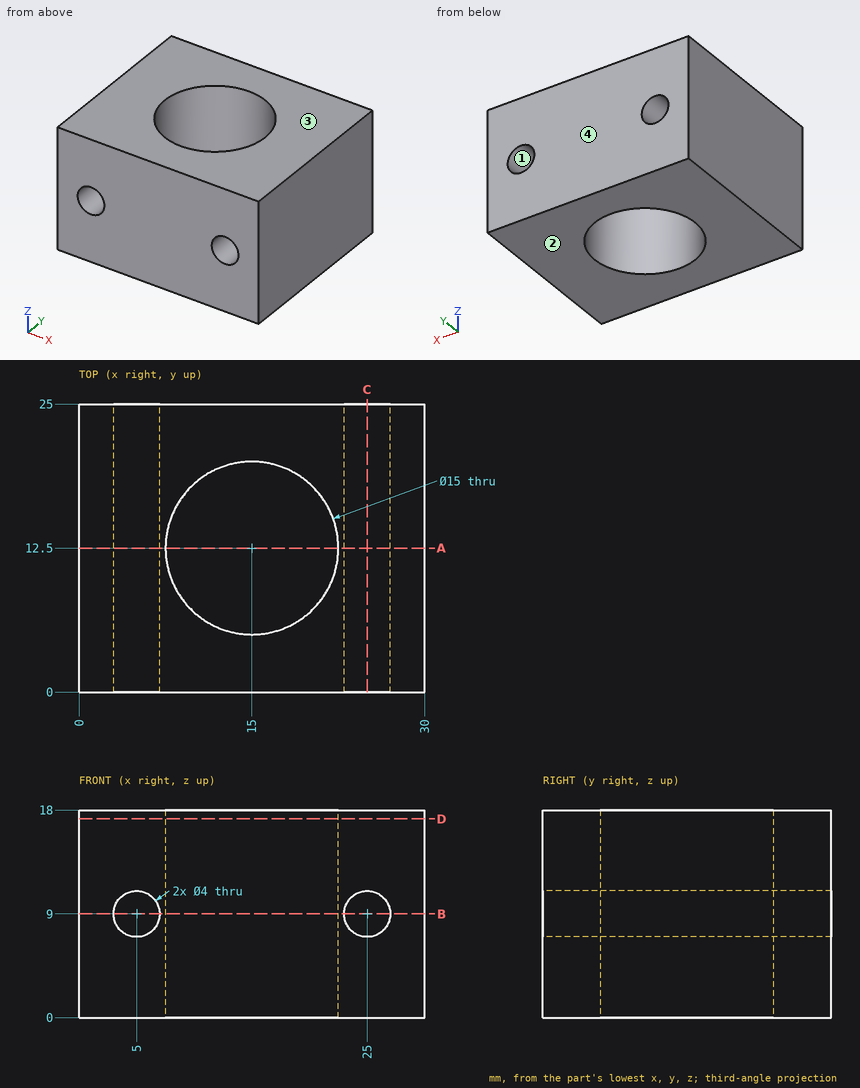
Design review of the part shown in the three views and the two pictorial views. Dimensions are in mm from the part's minimum x, y and z. Coordinates: 2 decimals unless noted, no trailing zeros. Loops run counter-clockwise (first coordinate to the right, second up) from the corner with the lowest first, then second, coordinate; pieces in that order, holes last. Notation, with made-up numbers: (42, 75) - (87, 75) arc R19 ccw to (87, 106) - close; hole circle Ø2 at (-39, 40.5). An arc over 180 degrees is marked (long way). Use a Markdown table: item, result. Add a question column.
Item 1: We need section B-B (z = 9). Give the boundary of the cut face in (x, y), and give its area (3 significant figures).
Item 2: For line 1 (Y direction, x = 15, z = 5.75); line 2 (Z direction, x = 25, y = 7.5); line 3 (X direction, y = 14.25, z = 9), list the stretches that pass through material, from the lowest coordinate up.
Item 3: Mouldability with a two-part tool opening along Z and no side actions: class the marked faces 1, 2, 3 and 4 as pulls with the +Z half, pulls with the -Z half, needs draft (parallel to the pull), parting line crosses it, or undercut.
Item 4: We need section D-D (z = 17.25). Give the boundary of the cut face in (x, y), and give its area (3 significant figures).
Item 5: We need section C-C (x = 25). Give the boundary of the cut face in (y, z), and give its area (3 significant figures).
Item 6: We need section A-A (y = 12.5). Give the boundary of the cut face in (x, z), and give its area (3 significant figures).
Results list:
| question | item | result |
|---|---|---|
| 1 | outline | (0, 0) - (3, 0) - (3, 25) - (0, 25) - close; (7, 0) - (23, 0) - (23, 25) - (7, 25) - close; (27, 0) - (30, 0) - (30, 25) - (27, 25) - close; hole circle Ø15 at (15, 12.5) |
| 1 | area | 373 mm^2 |
| 2 | line 1 | y = 0 to 5, 20 to 25 |
| 2 | line 2 | z = 0 to 7, 11 to 18 |
| 2 | line 3 | x = 0 to 3, 7 to 7.71, 22.29 to 23, 27 to 30 |
| 3 | face 1 | undercut |
| 3 | face 2 | pulls with the -Z half |
| 3 | face 3 | pulls with the +Z half |
| 3 | face 4 | needs draft |
| 4 | outline | (0, 0) - (30, 0) - (30, 25) - (0, 25) - close; hole circle Ø15 at (15, 12.5) |
| 4 | area | 573 mm^2 |
| 5 | outline | (0, 0) - (25, 0) - (25, 7) - (0, 7) - close; (0, 11) - (25, 11) - (25, 18) - (0, 18) - close |
| 5 | area | 350 mm^2 |
| 6 | outline | (0, 0) - (7.5, 0) - (7.5, 18) - (0, 18) - close; (22.5, 0) - (30, 0) - (30, 18) - (22.5, 18) - close; hole circle Ø4 at (5, 9); hole circle Ø4 at (25, 9) |
| 6 | area | 245 mm^2 |
